Geometry check sheet. Reference: the model listing, model coordinates, mm. Face numbers are marked on the shaded views. Give positions to 0.01 mm unless a question says otherwise; leave off trailing zeros. Write each loop counter-clockwise with the first axis right and the second up, starting at its lowest first coordinate (ties: lowest second). Pieces come first, ordered by that corner, then holes. Notation, with made-up numbers: M -23.75,84.25 L 24.25,84.25 A26 ccw 24.25,122.25 Z; hole C 1,28.5 d7. An arc over 180 degrees is marked long. One line per item, written item: value. Start each with the question number.
1. Gauge pin test, flat ends, axial feed: pin 1 (3 mm diameter, centred on x = 0, z = 0, fed in from -Y); pin 2 (2 mm diameter, centred on x = -29, y = 4, fed in from -Z); pin 3 (2.5 mm diameter, centred on y = 3, z = -5, fed in from +X). Record the tip position at first contact, or that the pin passes through.
2. Scan lines: line 1 (X direction, y = 0.75, z = 18); line 2 (X direction, y = 1.25, z = 55.5); line 3 (X direction, y = 4.15, z = 61). Record each from-to range of solid material in increasing order.
3. Cross-section at C-C on z = 9. Record the cut outline in (x, y), then the cut area to 3 significant figures.
4. Cross-section at D-D on x = 0. Count the separate pieces of the cut face and the enclosed holes in it, then the cut area to 3 significant figures.
5. Cross-section at B-B on z = 18. Record the cut outline in (x, y), then the cut area to 3 significant figures.
6. Release check for a two-part mould opening along X. For the marked faces 1 and 2 record: pulls with the +X half, pulls with the -X half, needs draft (parallel to the pull), parting line crosses it, or undercut.
7. Cross-section at A-A on x = -46. Record the cut outline in (y, z), then the cut area to 3 significant figures.
from build123d import *

# Parameters (mm, degrees)
SKETCH1_R           = 1.55
SKETCH1_R_2         = 2.55
BOSS_EXTRUDE1_DEPTH = 5
CUT_EXTRUDE1_DEPTH  = 2


with BuildPart() as part:
    # Sketch1 → Boss-Extrude1 (new body)
    with BuildSketch(Plane(origin=(0, 0, 0), x_dir=(1, 0, 0), z_dir=(0, 1, 0))):
        with BuildLine():
            Line((-13.25, 3), (-49, 3))
            ThreePointArc((-49, 3), (-52, 0), (-49, -3))
            Line((-49, -3), (-23.25, -3))
            ThreePointArc((-23.25, -3), (-16.178932188, -5.928932188), (-13.25, -13))
            Line((-13.25, -13), (-13.25, -71.173549983))
            ThreePointArc((-13.25, -71.173549983), (-12.371320344, -73.294870327), (-10.25, -74.173549983))
            Line((-10.25, -74.173549983), (10.25, -74.173549983))
            ThreePointArc((10.25, -74.173549983), (12.371320344, -73.294870327), (13.25, -71.173549983))
            Line((13.25, -71.173549983), (13.25, -13))
            ThreePointArc((13.25, -13), (16.178932188, -5.928932188), (23.25, -3))
            Line((23.25, -3), (49, -3))
            ThreePointArc((49, -3), (52, 0), (49, 3))
            Line((49, 3), (13.25, 3))
            Line((13.25, 3), (13.25, 9))
            ThreePointArc((13.25, 9), (12.371320344, 11.121320344), (10.25, 12))
            Line((10.25, 12), (-10.25, 12))
            ThreePointArc((-10.25, 12), (-12.371320344, 11.121320344), (-13.25, 9))
            Line((-13.25, 9), (-13.25, 3))
        make_face()
        with Locations(Location((-9, -45, 0), (0, 0, 270))):
            Circle(SKETCH1_R, mode=Mode.SUBTRACT)
        with Locations(Location((-9, -36, 0), (0, 0, 270))):
            Circle(SKETCH1_R, mode=Mode.SUBTRACT)
        with BuildLine():
            ThreePointArc((0, -46.55), (-1.55, -45), (0, -43.45))
            ThreePointArc((0, -43.45), (1.55, -45), (0, -46.55))
        make_face(mode=Mode.SUBTRACT)
        with Locations(Location((9, -45, 0), (0, 0, 270))):
            Circle(SKETCH1_R, mode=Mode.SUBTRACT)
        with BuildLine():
            ThreePointArc((0, -37.55), (-1.55, -36), (0, -34.45))
            ThreePointArc((0, -34.45), (1.55, -36), (0, -37.55))
        make_face(mode=Mode.SUBTRACT)
        with Locations(Location((9, -36, 0), (0, 0, 270))):
            Circle(SKETCH1_R, mode=Mode.SUBTRACT)
        with Locations(Location((-9, -27, 0), (0, 0, 270))):
            Circle(SKETCH1_R, mode=Mode.SUBTRACT)
        with Locations(Location((-9, -18, 0), (0, 0, 270))):
            Circle(SKETCH1_R, mode=Mode.SUBTRACT)
        with Locations(Location((-46, 0, 0), (0, 0, 270))):
            Circle(SKETCH1_R, mode=Mode.SUBTRACT)
        with BuildLine():
            ThreePointArc((0, -10.55), (-1.55, -9), (0, -7.45))
            ThreePointArc((0, -7.45), (1.55, -9), (0, -10.55))
        make_face(mode=Mode.SUBTRACT)
        with Locations(Location((-9, 0, 0), (0, 0, 270))):
            Circle(SKETCH1_R, mode=Mode.SUBTRACT)
        with BuildLine():
            ThreePointArc((0, -28.55), (-1.55, -27), (0, -25.45))
            ThreePointArc((0, -25.45), (1.55, -27), (0, -28.55))
        make_face(mode=Mode.SUBTRACT)
        with Locations(Location((9, -27, 0), (0, 0, 270))):
            Circle(SKETCH1_R, mode=Mode.SUBTRACT)
        with BuildLine():
            ThreePointArc((0, -19.55), (-1.55, -18), (0, -16.45))
            ThreePointArc((0, -16.45), (1.55, -18), (0, -19.55))
        make_face(mode=Mode.SUBTRACT)
        with Locations(Location((9, -18, 0), (0, 0, 270))):
            Circle(SKETCH1_R, mode=Mode.SUBTRACT)
        with BuildLine():
            ThreePointArc((0, -2.55), (-2.55, 0), (0, 2.55))
            ThreePointArc((0, 2.55), (2.55, 0), (0, -2.55))
        make_face(mode=Mode.SUBTRACT)
        with Locations(Location((9, 0, 0), (0, 0, 270))):
            Circle(SKETCH1_R, mode=Mode.SUBTRACT)
        with Locations(Location((0, 9, 0), (0, 0, 270))):
            Circle(SKETCH1_R, mode=Mode.SUBTRACT)
        with Locations(Location((46, 0, 0), (0, 0, 270))):
            Circle(SKETCH1_R, mode=Mode.SUBTRACT)
        with Locations(Location((0, -61, 0), (0, 0, 270))):
            Circle(SKETCH1_R_2, mode=Mode.SUBTRACT)
    extrude(amount=BOSS_EXTRUDE1_DEPTH)

    # Sketch2 → Cut-Extrude1 (cut)
    with BuildSketch(Plane.XZ):
        with BuildLine():
            Line((-11.5, 70.5), (-11.5, 51.5))
            ThreePointArc((-11.5, 51.5), (-10.914213562, 50.085786438), (-9.5, 49.5))
            Line((-9.5, 49.5), (9.5, 49.5))
            ThreePointArc((9.5, 49.5), (10.914213562, 50.085786438), (11.5, 51.5))
            Line((11.5, 51.5), (11.5, 70.5))
            ThreePointArc((11.5, 70.5), (10.914213562, 71.914213562), (9.5, 72.5))
            Line((9.5, 72.5), (-9.5, 72.5))
            ThreePointArc((-9.5, 72.5), (-10.914213562, 71.914213562), (-11.5, 70.5))
        make_face()
    extrude(amount=-CUT_EXTRUDE1_DEPTH, mode=Mode.SUBTRACT)


solid = part.part
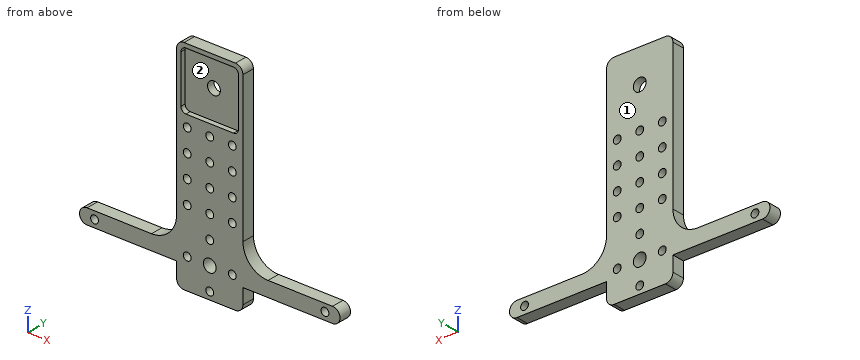
Report:
1. pin 1: passes through
1. pin 2: stops at z = -3
1. pin 3: stops at x = 13.25
2. line 1: x = -13.25 to -10.55, -7.45 to -1.55, 1.55 to 7.45, 10.55 to 13.25
2. line 2: x = -13.25 to -11.5, 11.5 to 13.25
2. line 3: x = -13.25 to -2.55, 2.55 to 13.25
3. outline: M -14.08,0 L -1.55,0 L -1.55,5 L -14.08,5 Z; M 1.55,0 L 14.08,0 L 14.08,5 L 1.55,5 Z
3. area: 125 mm^2
4. separate pieces: 9
4. enclosed holes: 0
4. area: 251 mm^2
5. outline: M -13.25,0 L -10.55,0 L -10.55,5 L -13.25,5 Z; M -7.45,0 L -1.55,0 L -1.55,5 L -7.45,5 Z; M 1.55,0 L 7.45,0 L 7.45,5 L 1.55,5 Z; M 10.55,0 L 13.25,0 L 13.25,5 L 10.55,5 Z
5. area: 86.0 mm^2
6. face 1: needs draft
6. face 2: undercut
7. outline: M 0,-3 L 5,-3 L 5,-1.55 L 0,-1.55 Z; M 0,1.55 L 5,1.55 L 5,3 L 0,3 Z
7. area: 14.5 mm^2
